Geometry: final body of the model. Coordinates: model frame, mm. Round coordinates to 2 decimals unless told otherwise and drop trailing zeros. Loops run counter-clockwise (first coordinate to the right, second up) from the corner with the lowest first, then second, coordinate; pieces in that order, holes last. Notation, with made-up numbers: (75, 9) - (91, 9) arc R26 ccw to (91, 34) - close; hole circle Ø3 at (26.5, -22.5). An arc over 180 degrees is marked (long way). Answer as CSV lines item,"result".
from build123d import *

# Parameters (mm, degrees)
RESSALTO_EXTRUS_O1_DEPTH = 105
FILETE1_R                = 0.5


with BuildPart() as part:
    # Esboço1 → Ressalto-extrusão1 (new body)
    with BuildSketch(Plane.XY.offset(135)):
        Polygon((-55.002122675, 2.886751346), (-57.502122675, 1.443375673), (-57.502122675, -1.443375673), (-55.002122675, -2.886751346), (-52.502122675, -1.443375673), (-52.502122675, 1.443375673), align=None)
    extrude(amount=-RESSALTO_EXTRUS_O1_DEPTH)

    # Filete1
    filete1_edges = [part.edges().sort_by_distance(p)[0] for p in [
        (-57.502122675, 0, 30),
        (-56.252122675, -2.165063509, 30),
        (-53.752122675, -2.165063509, 30),
        (-52.502122675, 0, 30),
        (-53.752122675, 2.165063509, 30),
        (-52.502122675, 0, 135),
        (-53.752122675, -2.165063509, 135),
        (-56.252122675, -2.165063509, 135),
        (-57.502122675, 0, 135),
        (-56.252122675, 2.165063509, 135),
        (-53.752122675, 2.165063509, 135),
        (-56.252122675, 2.165063509, 30),
    ]]
    fillet(filete1_edges, radius=FILETE1_R)


solid = part.part
(1) Material intervals for line 1 along Z through (x, y) = (-55.2, -2.3); line 2 along Y through (x, z) = (-56.1, 76); line 3 along Y through (x, z) = (-54.4, 121), sorted ascending.
Findings below:
line 1,"30.01 to 134.99"
line 2,"-2.25 to 2.25"
line 3,"-2.54 to 2.54"
(2) Pin query (flat end, axial travel): P1, Ø1, axis at x = -53, z = 105, coming from the -Y side; P2, Ø2, axis at x = -54.5, z = 112.5, coming from the -Y side. Return the tip coordinate at first contact, or that it passes through.
Findings below:
P1,"y = -2.02"
P2,"y = -2.89"
(3) Section A-A (z = 91.5). Output: boundary loops of the cut face in (x, y).
Findings below:
outline,"(-57.5, -1.44) - (-55, -2.89) - (-52.5, -1.44) - (-52.5, 1.44) - (-55, 2.89) - (-57.5, 1.44) - close"
